```python
from build123d import *

# Parameters (mm, degrees)
SKETCH_1_W          = 45
SKETCH_1_H          = 45
EXTRUDE_1_DEPTH     = 15
SKETCH_2_W          = 4
SKETCH_2_H          = 8
EXTRUDE_2_DEPTH     = 3
SKETCH_3_R          = 6.25
CUT_EXTRUDE_1_DEPTH = 16
SKETCH_4_R          = 10
CUT_EXTRUDE_2_DEPTH = 9
CUT_EXTRUDE_3_DEPTH = 7
SKETCH_6_R          = 5.5
CUT_EXTRUDE_4_DEPTH = 2
FILLET_1_R          = 2


with BuildPart() as part:
    # Эскиз1 → Бобышка-Вытянуть1 (new body)
    with BuildSketch(Plane(origin=(0, 0, 0), x_dir=(1, 0, 0), z_dir=(0, 1, 0))):
        Rectangle(SKETCH_1_W, SKETCH_1_H)
    extrude(amount=EXTRUDE_1_DEPTH)

    # Эскиз2 → Бобышка-Вытянуть2 (add)
    with BuildSketch(Plane(origin=(0, 15, 0), x_dir=(1, 0, 0), z_dir=(0, 1, 0))):
        with Locations((-20.5, 0)):
            Rectangle(SKETCH_2_W, SKETCH_2_H)
        with Locations((20.5, 0)):
            Rectangle(SKETCH_2_W, SKETCH_2_H)
    extrude(amount=EXTRUDE_2_DEPTH)

    # Эскиз3 → Вырез-Вытянуть1 (cut, through all)
    with BuildSketch(Plane(origin=(0, 15, 0), x_dir=(1, 0, 0), z_dir=(0, 1, 0))):
        with Locations(Location((0, 0, 0), (0, 0, 270))):  # turned: the seam where the file's is
            Circle(SKETCH_3_R)
        with BuildLine():
            Line((-3.25, -22.5), (-3.25, -16))
            ThreePointArc((-3.25, -16), (0, -12.75), (3.25, -16))
            Line((3.25, -16), (3.25, -22.5))
            Line((3.25, -22.5), (-3.25, -22.5))
        make_face()
        with BuildLine():
            Line((3.25, 16), (3.25, 22.5))
            Line((3.25, 22.5), (-3.25, 22.5))
            Line((-3.25, 22.5), (-3.25, 16))
            ThreePointArc((-3.25, 16), (0, 12.75), (3.25, 16))
        make_face()
    extrude(amount=-CUT_EXTRUDE_1_DEPTH, mode=Mode.SUBTRACT)

    # Эскиз4 → Вырез-Вытянуть2 (cut)
    with BuildSketch(Plane.XZ):
        with Locations(Location((0, 0, 0), (0, 0, 270))):  # turned: the seam where the file's is
            Circle(SKETCH_4_R)
    extrude(amount=-CUT_EXTRUDE_2_DEPTH, mode=Mode.SUBTRACT)

    # Эскиз5 → Вырез-Вытянуть3 (cut)
    with BuildSketch(Plane(origin=(0, 15, 0), x_dir=(1, 0, 0), z_dir=(0, 1, 0))):
        with BuildLine():
            Line((-5.5, -22.5), (-5.5, -16))
            ThreePointArc((-5.5, -16), (0, -10.5), (5.5, -16))
            Line((5.5, -16), (5.5, -22.5))
            Line((5.5, -22.5), (-5.5, -22.5))
        make_face()
        with BuildLine():
            Line((5.5, 16), (5.5, 22.5))
            Line((5.5, 22.5), (-5.5, 22.5))
            Line((-5.5, 22.5), (-5.5, 16))
            ThreePointArc((-5.5, 16), (0, 10.5), (5.5, 16))
        make_face()
    extrude(amount=-CUT_EXTRUDE_3_DEPTH, mode=Mode.SUBTRACT)

    # Эскиз6 → Вырез-Вытянуть4 (cut)
    with BuildSketch(Plane(origin=(0, 8, 0), x_dir=(1, 0, 0), z_dir=(0, 1, 0))):
        with Locations((0, -16)):
            Circle(SKETCH_6_R)
        with Locations((0, 16)):
            Circle(SKETCH_6_R)
    extrude(amount=-CUT_EXTRUDE_4_DEPTH, mode=Mode.SUBTRACT)

    # Скругление1
    fillet_1_edges = [part.edges().sort_by_distance(p)[0] for p in [
        (-22.5, 7.5, -22.5),
        (22.5, 7.5, -22.5),
        (22.5, 7.5, 22.5),
        (-22.5, 7.5, 22.5),
    ]]
    fillet(fillet_1_edges, radius=FILLET_1_R)


solid = part.part
```
Geometry check sheet. Reference: the model listing, model coordinates, mm. A direction names the side the tool comes from. Coordinates: 2 decimals unless noted, no trailing zeros. Write each loop counter-clockwise with the first axis right and the second up, starting at its lowest first coordinate (ties: lowest second). Pieces come first, ordered by that corner, then holes. Notation, with made-up numbers: (80, 85) -> (133, 85) arc R16 cw to (133, 110) -> close; hole circle Ø3 at (20.25, 24). An arc over 180 degrees is marked (long way). Use CSV: the item, a comma, the result in double quotes. Start each with the question number.
Item 1: Set-up check for faces 1 (the flat face through (5, 9, -4)), 2 (the flat face through (-5.5, 12, -19)), 3 (the flat face through (-5.5, 12, 19)), 4 (the flat face through (3.25, 3, 19)), 5 (the flat face through (-21, 16, -4)): record each of +Z, -Z, +X, -X, +Y, -Y from which the full face is reachable in a straight line by a thin tool's end or side.
Item 2: Thickness scan on line 1 (X direction, y = 9.5, z = 16); line 2 (X direction, y = 6.5, z = 0); line 3 (Y direction, x = 7, z = 6). Record the ranges inside material, lowest first.
Item 3: Cross-section at D-D, the plane x = -8.5. Record the cut outline in (y, z), plus the area to 3 significant figures.
Item 4: Cross-section at C-C, the plane y = 17.25. Record the cut outline in (x, z).
Item 5: Depth check by flat-ended pin: pin 1 Ø2 at (x, y) = (-4, 13.5) entering from +Z; pin 2 Ø0.9 at (x, y) = (21, 16.5) entering from +Z; pin 3 Ø1.1 at (x, z) = (-4.5, 20) entering from +Y. Enter the tip coordinate at first touch or a pass-through.
Item 6: Cross-section at A-A, the plane y = 13.75. Record the cut outline in (x, z), plus the area to 3 significant figures.
Item 7: Mould release check, pull along X, two halves, no side actions. Record for faces 6 (the flat face through (18.5, 16, 0)), 7 (the flat face through (20, 16, -4)), 8 (the cylindrical face through (-21.93, 7.6, -21.9)): released by +X, released by -X, zero draft, split by the parting line, or undercut.
Item 8: Cross-section at B-B, the plane z = 5. Record the cut outline in (x, y).
Answers:
1,face 1,"-Y"
1,face 2,"-Z, +Y"
1,face 3,"+Z, +Y"
1,face 4,"+Z, +Y, -Y"
1,face 5,"-Z, +X, -X, +Y"
2,line 1,"-22.5 to -5.5, 5.5 to 22.5"
2,line 2,"-22.5 to -10, 10 to 22.5"
2,line 3,"9 to 15"
3,outline,"(0, -22.5) -> (15, -22.5) -> (15, 22.5) -> (0, 22.5) -> (0, 5.27) -> (9, 5.27) -> (9, -5.27) -> (0, -5.27) -> close"
3,area,"580 mm^2"
4,outline,"(-22.5, -4) -> (-18.5, -4) -> (-18.5, 4) -> (-22.5, 4) -> close; (18.5, -4) -> (22.5, -4) -> (22.5, 4) -> (18.5, 4) -> close"
5,pin 1,"z = 13.71"
5,pin 2,"z = 4"
5,pin 3,"y = 8"
6,outline,"(-22.5, -20.5) arc R2 ccw to (-20.5, -22.5) -> (-5.5, -22.5) -> (-5.5, -16) arc R5.5 cw to (5.5, -16) -> (5.5, -22.5) -> (20.5, -22.5) arc R2 ccw to (22.5, -20.5) -> (22.5, 20.5) arc R2 ccw to (20.5, 22.5) -> (5.5, 22.5) -> (5.5, 16) arc R5.5 cw to (-5.5, 16) -> (-5.5, 22.5) -> (-20.5, 22.5) arc R2 ccw to (-22.5, 20.5) -> close; hole circle Ø12.5 at (0, 0)"
6,area,"1,660 mm^2"
7,face 6,"undercut"
7,face 7,"zero draft"
7,face 8,"released by -X"
8,outline,"(-22.5, 0) -> (-8.66, 0) -> (-8.66, 9) -> (-3.75, 9) -> (-3.75, 15) -> (-22.5, 15) -> close; (3.75, 9) -> (8.66, 9) -> (8.66, 0) -> (22.5, 0) -> (22.5, 15) -> (3.75, 15) -> close"
